Input: part model. Units: mm. Frame: model coordinates. Face numbers are marked on the shaded views. A direction names the side the tool comes from. Coordinates: 2 decimals unless noted, no trailing zeros. Order: outer loops, then holes, each group sorted by start corner. A loop starts at its lowest first (then second) coordinate and runs counter-clockwise, first axis right, second up. Notation, with made-up numbers: (80, -24.75) -> (87, -24.75) arc R13 ccw to (87, -3.75) -> close; hole circle Ø2 at (0.5, -5.75). An arc over 180 degrees is marked (long way). Use one line per item in the form item = value. Start each with the question number.
1) Ray query, line 1 along X through (y, z) = (-6, 6.75); line 2 along X through (y, z) = (-3.25, 1.5); line 3 along Z through (x, y) = (-7.5, -0.75). Return the intervals inside material, ascending.
2) Pin query (flat end, axial travel): pin 1 (0.8 mm diameter, centred on x = -11, y = -7.5, fed in from +Z); pin 2 (3 mm diameter, centred on y = -4, z = -2, fed in from +X); pin 3 (1 mm diameter, centred on y = -1.5, z = 5.5, fed in from -X). Return the tip coordinate at first contact, or that it passes through.
3) Access query for the marked faces 1 and 2. Directions: +Z, -Z, +X, -X, +Y, -Y. A direction counts if a zero-diameter tool reaches every point of the face in a straight line with its end or side. Return the directions, or none.
4) Draft query along Z for the marked faces 3, 4, 5 and 6. Return one class per face: pulls with the +Z half, pulls with the -Z half, needs draft (parallel to the pull), parting line crosses it, or undercut.
5) Section query B-B on x = 6. Output: boundary loops of the cut face in (y, z), then the cut area to 3 significant figures.
6) Section query A-A on z = 3. Output: boundary loops of the cut face in (x, y).
7) Section query C-C on y = -8.75. Output: boundary loops of the cut face in (x, z) (3 decimals).
8) Section query D-D on z = 0. Output: boundary loops of the cut face in (x, y), then the cut area to 3 significant figures.
from build123d import *

# Parameters (mm, degrees)
F1_DEPTH = 12.7
F3_DEPTH = 12.7
F4_DEPTH = 0.254
F5_R     = 5.715
F5_R_2   = 5.0844343855
F6_DEPTH = 0.254


with BuildPart() as f1:
    # F0 (on Front) → F1 (new body)
    with BuildSketch(Plane.XZ):
        with BuildLine():
            Line((-1.1751782149, -4.8178826279), (-1.1751782149, 1.5321173721))
            ThreePointArc((-1.1751782149, 1.5321173721), (-3.0350501544, -2.9580106884), (-7.5251782149, -4.8178826279))
            Line((-7.5251782149, -4.8178826279), (-1.1751782149, -4.8178826279))
        make_face()
        with BuildLine():
            Line((-13.2001757149, 2.2071198721), (-13.8751782149, 1.5321173721))
            Line((-13.8751782149, 1.5321173721), (-13.2401782149, 1.5321173721))
            ThreePointArc((-13.2401782149, 1.5321173721), (-13.2301688246, 1.8702107672), (-13.2001757149, 2.2071198721))
        make_face()
        with BuildLine():
            Line((-13.2401782149, 1.5321173721), (-13.8751782149, 1.5321173721))
            Line((-13.8751782149, 1.5321173721), (-13.2001757149, 0.8571148721))
            ThreePointArc((-13.2001757149, 0.8571148721), (-13.2301688246, 1.1940239771), (-13.2401782149, 1.5321173721))
        make_face()
        with BuildLine():
            Line((-8.2001807149, -4.1428801279), (-7.5251782149, -4.8178826279))
            Line((-7.5251782149, -4.8178826279), (-7.5251782149, -4.1828826279))
            ThreePointArc((-7.5251782149, -4.1828826279), (-7.8632716099, -4.1728732375), (-8.2001807149, -4.1428801279))
        make_face()
        with BuildLine():
            Line((-7.5251782149, -4.1828826279), (-7.5251782149, -4.8178826279))
            Line((-7.5251782149, -4.8178826279), (-6.8501757149, -4.1428801279))
            ThreePointArc((-6.8501757149, -4.1428801279), (-7.1870848199, -4.1728732375), (-7.5251782149, -4.1828826279))
        make_face()
        with BuildLine():
            Line((-6.8501757149, 7.2071148721), (-7.5251782149, 7.8821173721))
            Line((-7.5251782149, 7.8821173721), (-7.5251782149, 7.2471173721))
            ThreePointArc((-7.5251782149, 7.2471173721), (-7.1870848199, 7.2371079818), (-6.8501757149, 7.2071148721))
        make_face()
        with BuildLine():
            Line((-7.5251782149, 7.2471173721), (-7.5251782149, 7.8821173721))
            Line((-7.5251782149, 7.8821173721), (-8.2001807149, 7.2071148721))
            ThreePointArc((-8.2001807149, 7.2071148721), (-7.8632716099, 7.2371079818), (-7.5251782149, 7.2471173721))
        make_face()
        with BuildLine():
            ThreePointArc((-1.1751782149, 1.5321173721), (-3.0350501544, 6.0222454327), (-7.5251782149, 7.8821173721))
            Line((-7.5251782149, 7.8821173721), (-6.8501757149, 7.2071148721))
            ThreePointArc((-6.8501757149, 7.2071148721), (-5.9783416171, 7.0338008908), (-5.1439282149, 6.7273915167))
            ThreePointArc((-5.1439282149, 6.7273915167), (-3.4840629604, 5.5732326266), (-2.3299040703, 3.9133673721))
            ThreePointArc((-2.3299040703, 3.9133673721), (-2.0234946962, 3.07895397), (-1.8501807149, 2.2071198721))
            Line((-1.8501807149, 2.2071198721), (-1.1751782149, 1.5321173721))
        make_face()
        with BuildLine():
            Line((-8.2001807149, 7.2071148721), (-7.5251782149, 7.8821173721))
            ThreePointArc((-7.5251782149, 7.8821173721), (-12.0153062754, 6.0222454327), (-13.8751782149, 1.5321173721))
            Line((-13.8751782149, 1.5321173721), (-13.2001757149, 2.2071198721))
            ThreePointArc((-13.2001757149, 2.2071198721), (-13.0268617336, 3.07895397), (-12.7204523595, 3.9133673721))
            ThreePointArc((-12.7204523595, 3.9133673721), (-11.5662934694, 5.5732326266), (-9.9064282149, 6.7273915167))
            ThreePointArc((-9.9064282149, 6.7273915167), (-9.0720148127, 7.0338008908), (-8.2001807149, 7.2071148721))
        make_face()
        with BuildLine():
            Line((-13.2001757149, 0.8571148721), (-13.8751782149, 1.5321173721))
            ThreePointArc((-13.8751782149, 1.5321173721), (-12.0153062754, -2.9580106884), (-7.5251782149, -4.8178826279))
            Line((-7.5251782149, -4.8178826279), (-8.2001807149, -4.1428801279))
            ThreePointArc((-8.2001807149, -4.1428801279), (-9.0720148127, -3.9695661465), (-9.9064282149, -3.6631567725))
            ThreePointArc((-9.9064282149, -3.6631567725), (-11.5662934694, -2.5089978823), (-12.7204523595, -0.8491326279))
            ThreePointArc((-12.7204523595, -0.8491326279), (-13.0268617336, -0.0147192257), (-13.2001757149, 0.8571148721))
        make_face()
        with BuildLine():
            ThreePointArc((-7.5251782149, -4.8178826279), (-3.0350501544, -2.9580106884), (-1.1751782149, 1.5321173721))
            Line((-1.1751782149, 1.5321173721), (-1.8501807149, 0.8571148721))
            ThreePointArc((-1.8501807149, 0.8571148721), (-2.0234946962, -0.0147192257), (-2.3299040703, -0.8491326279))
            ThreePointArc((-2.3299040703, -0.8491326279), (-3.4840629604, -2.5089978823), (-5.1439282149, -3.6631567725))
            ThreePointArc((-5.1439282149, -3.6631567725), (-5.9783416171, -3.9695661465), (-6.8501757149, -4.1428801279))
            Line((-6.8501757149, -4.1428801279), (-7.5251782149, -4.8178826279))
        make_face()
        with BuildLine():
            Line((-9.9064282149, 5.5008673721), (-9.9064282149, 6.7273915167))
            ThreePointArc((-9.9064282149, 6.7273915167), (-11.5662934694, 5.5732326266), (-12.7204523595, 3.9133673721))
            Line((-12.7204523595, 3.9133673721), (-11.4939282149, 3.9133673721))
            Line((-11.4939282149, 3.9133673721), (-10.7001782149, 4.7071173721))
            Line((-10.7001782149, 4.7071173721), (-9.9064282149, 5.5008673721))
        make_face()
        Polygon((-9.9064282149, 3.9133673721), (-9.9064282149, 5.5008673721), (-10.7001782149, 4.7071173721), align=None)
        Polygon((-10.7001782149, 4.7071173721), (-11.4939282149, 3.9133673721), (-9.9064282149, 3.9133673721), align=None)
        Polygon((-4.3501782149, 4.7071173721), (-5.1439282149, 5.5008673721), (-5.1439282149, 3.9133673721), align=None)
        with BuildLine():
            ThreePointArc((-2.3299040703, 3.9133673721), (-3.4840629604, 5.5732326266), (-5.1439282149, 6.7273915167))
            Line((-5.1439282149, 6.7273915167), (-5.1439282149, 5.5008673721))
            Line((-5.1439282149, 5.5008673721), (-4.3501782149, 4.7071173721))
            Line((-4.3501782149, 4.7071173721), (-3.5564282149, 3.9133673721))
            Line((-3.5564282149, 3.9133673721), (-2.3299040703, 3.9133673721))
        make_face()
        Polygon((-5.1439282149, 3.9133673721), (-3.5564282149, 3.9133673721), (-4.3501782149, 4.7071173721), align=None)
        with BuildLine():
            ThreePointArc((-5.1439282149, -3.6631567725), (-3.4840629604, -2.5089978823), (-2.3299040703, -0.8491326279))
            Line((-2.3299040703, -0.8491326279), (-3.5564282149, -0.8491326279))
            Line((-3.5564282149, -0.8491326279), (-4.3501782149, -1.6428826279))
            Line((-4.3501782149, -1.6428826279), (-5.1439282149, -2.4366326279))
            Line((-5.1439282149, -2.4366326279), (-5.1439282149, -3.6631567725))
        make_face()
        Polygon((-4.3501782149, -1.6428826279), (-3.5564282149, -0.8491326279), (-5.1439282149, -0.8491326279), align=None)
        Polygon((-5.1439282149, -0.8491326279), (-5.1439282149, -2.4366326279), (-4.3501782149, -1.6428826279), align=None)
        with BuildLine():
            Line((-11.4939282149, -0.8491326279), (-12.7204523595, -0.8491326279))
            ThreePointArc((-12.7204523595, -0.8491326279), (-11.5662934694, -2.5089978823), (-9.9064282149, -3.6631567725))
            Line((-9.9064282149, -3.6631567725), (-9.9064282149, -2.4366326279))
            Line((-9.9064282149, -2.4366326279), (-10.7001782149, -1.6428826279))
            Line((-10.7001782149, -1.6428826279), (-11.4939282149, -0.8491326279))
        make_face()
        Polygon((-10.7001782149, -1.6428826279), (-9.9064282149, -2.4366326279), (-9.9064282149, -0.8491326279), align=None)
        Polygon((-9.9064282149, -0.8491326279), (-11.4939282149, -0.8491326279), (-10.7001782149, -1.6428826279), align=None)
        with BuildLine():
            Line((-1.8101782149, 1.5321173721), (-1.1751782149, 1.5321173721))
            Line((-1.1751782149, 1.5321173721), (-1.8501807149, 2.2071198721))
            ThreePointArc((-1.8501807149, 2.2071198721), (-1.8201876053, 1.8702107672), (-1.8101782149, 1.5321173721))
        make_face()
        with BuildLine():
            Line((-1.8501807149, 0.8571148721), (-1.1751782149, 1.5321173721))
            Line((-1.1751782149, 1.5321173721), (-1.8101782149, 1.5321173721))
            ThreePointArc((-1.8101782149, 1.5321173721), (-1.8201876053, 1.1940239771), (-1.8501807149, 0.8571148721))
        make_face()
        with BuildLine():
            Line((-1.1751782149, 7.8821173721), (-7.5251782149, 7.8821173721))
            ThreePointArc((-7.5251782149, 7.8821173721), (-3.0350501544, 6.0222454327), (-1.1751782149, 1.5321173721))
            Line((-1.1751782149, 1.5321173721), (-1.1751782149, 7.8821173721))
        make_face()
        Polygon((11.5248217851, 7.8821173721), (-1.1751782149, 7.8821173721), (-1.1751782149, 1.5321173721), (-1.1751782149, -4.8178826279), (11.5248217851, -4.8178826279), align=None)
    extrude(amount=F1_DEPTH)

    # F2 (on face) → F3 (cut)
    with BuildSketch(Plane.XY.offset(7.8821173721)):
        with BuildLine():
            Line((11.5248217851, 0), (5.1748217851, 0))
            ThreePointArc((5.1748217851, 0), (9.6649498456, -1.8598719395), (11.5248217851, -6.35))
            Line((11.5248217851, -6.35), (11.5248217851, 0))
        make_face()
        with BuildLine():
            Line((11.5248217851, -12.7), (11.5248217851, -6.35))
            ThreePointArc((11.5248217851, -6.35), (9.6649498456, -10.8401280605), (5.1748217851, -12.7))
            Line((5.1748217851, -12.7), (11.5248217851, -12.7))
        make_face()
        with BuildLine():
            Line((5.1748217851, -11.4344343855), (5.1748217851, -1.2655656145))
            ThreePointArc((5.1748217851, -1.2655656145), (0.0903873996, -6.35), (5.1748217851, -11.4344343855))
        make_face()
        with BuildLine():
            ThreePointArc((10.2592561706, -6.35), (8.7700598176, -2.7547619675), (5.1748217851, -1.2655656145))
            Line((5.1748217851, -1.2655656145), (5.1748217851, -11.4344343855))
            ThreePointArc((5.1748217851, -11.4344343855), (8.7700598176, -9.9452380325), (10.2592561706, -6.35))
        make_face()
    extrude(amount=-F3_DEPTH, mode=Mode.SUBTRACT)

    # F2 (on face) → F4 (cut)
    with BuildSketch(Plane.XY.offset(7.8821173721)):
        with BuildLine():
            Line((5.1748217851, -1.2655656145), (5.1748217851, -0.635))
            ThreePointArc((5.1748217851, -0.635), (-0.5401782149, -6.35), (5.1748217851, -12.065))
            Line((5.1748217851, -12.065), (5.1748217851, -11.4344343855))
            ThreePointArc((5.1748217851, -11.4344343855), (0.0903873996, -6.35), (5.1748217851, -1.2655656145))
        make_face()
        with BuildLine():
            ThreePointArc((10.8898217851, -6.35), (9.2159370396, -2.3088847455), (5.1748217851, -0.635))
            Line((5.1748217851, -0.635), (5.1748217851, -1.2655656145))
            ThreePointArc((5.1748217851, -1.2655656145), (8.7700598176, -2.7547619675), (10.2592561706, -6.35))
            ThreePointArc((10.2592561706, -6.35), (8.7700598176, -9.9452380325), (5.1748217851, -11.4344343855))
            Line((5.1748217851, -11.4344343855), (5.1748217851, -12.065))
            ThreePointArc((5.1748217851, -12.065), (9.2159370396, -10.3911152545), (10.8898217851, -6.35))
        make_face()
    extrude(amount=-F4_DEPTH, mode=Mode.SUBTRACT)

    # F5 (on face) → F6 (cut)
    with BuildSketch(Plane(origin=(0, 0, -4.8178826279), x_dir=(1, 0, 0), z_dir=(0, 0, -1))):
        with Locations((5.1748217851, 6.35)):
            Circle(F5_R)
        with Locations((5.1748217851, 6.35)):
            Circle(F5_R_2, mode=Mode.SUBTRACT)
    extrude(amount=-F6_DEPTH, mode=Mode.SUBTRACT)


solid = f1.part
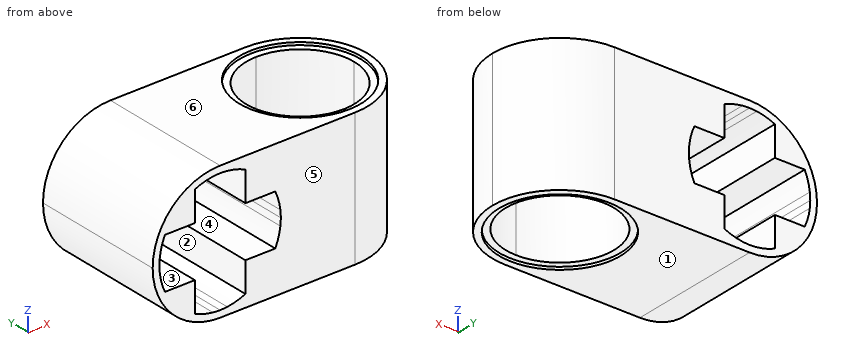
Answers below:
q1.line_1 = -11.14 to -9.86, -5.19 to 0.1, 10.25 to 11.52
q1.line_2 = -13.88 to -13.24, -1.81 to 1.14, 9.2 to 10.72
q1.line_3 = -4.82 to -4.18, 7.25 to 7.88
q2.pin_1 = 7.09
q2.pin_2 = 11.47
q2.pin_3 = -12.84
q3.face_1 = -Z, +X, -X, +Y, -Y
q3.face_2 = +Y, -Y
q4.face_3 = undercut
q4.face_4 = undercut
q4.face_5 = needs draft
q4.face_6 = pulls with the +Z half
q5.outline = (-12.65, -4.82) -> (-12.01, -4.82) -> (-12.01, -4.56) -> (-11.37, -4.56) -> (-11.37, 7.63) -> (-12.01, 7.63) -> (-12.01, 7.88) -> (-12.65, 7.88) -> close; (-1.33, -4.56) -> (-0.69, -4.56) -> (-0.69, -4.82) -> (-0.05, -4.82) -> (-0.05, 7.88) -> (-0.69, 7.88) -> (-0.69, 7.63) -> (-1.33, 7.63) -> close
q5.area = 31.8 mm^2
q6.outline = (-13.7, -12.7) -> (-13.05, -12.7) -> (-13.05, 0) -> (-13.7, 0) -> close; (-2, -12.7) -> (5.17, -12.7) arc R6.35 ccw to (5.17, 0) -> (-2, 0) -> close; hole circle Ø10.17 at (5.17, -6.35)
q7.outline = (-7.525, -4.818) -> (-0.012, -4.818) -> (-0.012, -4.564) -> (0.692, -4.564) -> (0.692, 7.628) -> (-0.012, 7.628) -> (-0.012, 7.882) -> (-7.525, 7.882) arc R6.35 ccw to start; (9.657, -4.564) -> (10.361, -4.564) -> (10.361, -4.818) -> (11.054, -4.818) -> (11.054, 7.882) -> (10.361, 7.882) -> (10.361, 7.628) -> (9.657, 7.628) -> close; hole (-12.72, -0.849) -> (-9.906, -0.849) -> (-9.906, -3.663) arc R5.715 ccw to (-5.144, -3.663) -> (-5.144, -0.849) -> (-2.33, -0.849) arc R5.715 ccw to (-2.33, 3.913) -> (-5.144, 3.913) -> (-5.144, 6.727) arc R5.715 ccw to (-9.906, 6.727) -> (-9.906, 3.913) -> (-12.72, 3.913) arc R5.715 ccw to start
q8.outline = (-13.69, -12.7) -> (-13.03, -12.7) -> (-13.03, 0) -> (-13.69, 0) -> close; (-2.02, -12.7) -> (5.17, -12.7) arc R6.35 ccw to (5.17, 0) -> (-2.02, 0) -> close; hole circle Ø10.17 at (5.17, -6.35)
q8.area = 81.8 mm^2
